Verification items for the finished model (mm, model axes). Face numbers are marked on the shaded views. A direction names the side the tool comes from. Coordinates: 2 decimals unless noted, no trailing zeros. Loops run counter-clockwise (first coordinate to the right, second up) from the corner with the lowest first, then second, coordinate; pieces in that order, holes last.
Q1. Sectioned sample at D-D (z = -3). Enter the section's corners in (x, y), then the cut area to 3 significant figures.
Q2. Sectioned sample at A-A (x = -40.5). Enter the section's corners in (y, z).
Q3. Access from +Z, -Z, +X, -X, +Y, -Y to the whole of each face (thin tool, end or side, straight path). Record for the marked faces 1, 2 and 3.
Q4. Sectioned sample at B-B (y = 0). Count the separate pieces of the cut face and the enclosed holes in it, then the cut area to 3 significant figures.
Q5. Sectioned sample at C-C (x = 44). Enter the section's corners in (y, z), then the cut area to 3 significant figures.
Q6. Go/stop test with flat-tipped pins: P1, Ø0.5, axis at y = -12, z = 1.5, coming from the +X side; P2, Ø23.5, axis at x = -36, y = -9.5, coming from the -Z side; P3, Ø5, axis at x = -40.5, z = -4, coming from the -Y side; P4, Ø4, axis at y = -8.5, z = -6.5, coming from the +X side. Record where each tip stops, or that it passes through.
Q7. Material ranges on probe 1 along Z at (x, y) = (-41, -22); probe 2 along Y at (x, z) = (11, -2.5); probe 3 along Y at (x, z) = (-40.5, 1.9), recorded low to high.
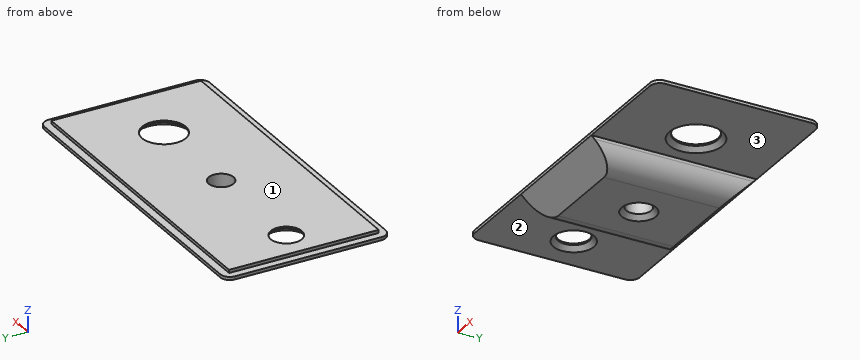
```python
from build123d import *

# Parameters (mm, degrees)
F0_W            = 106
F0_H            = 53
F1_DEPTH        = 1
F2_W            = 101
F2_H            = 48
F3_DEPTH        = 1
F4_R            = 3
F6_D            = 14
F6_CSINK_D      = 17
F6_CSINK_ANGLE  = 90
F7_D            = 10
F7_CSINK_D      = 13
F7_CSINK_ANGLE  = 90
F8_W            = 40
F8_H            = 53
F9_DEPTH        = 8
F11_D           = 8
F11_CSINK_D     = 11
F11_CSINK_ANGLE = 90
F12_SIZE        = 8
F13_R           = 7


with BuildPart() as f1:
    # F0 (on Top) → F1 (new body)
    with BuildSketch(Plane.XY):
        Rectangle(F0_W, F0_H)
    extrude(amount=F1_DEPTH)

    # F2 (on face) → F3 (join)
    with BuildSketch(Plane.XY.offset(1)):
        Rectangle(F2_W, F2_H)
    extrude(amount=F3_DEPTH)

    # F4
    f4_edges = [f1.edges().sort_by_distance(p)[0] for p in [
        (-53, -26.5, 0.5),
        (53, -26.5, 0.5),
        (53, 26.5, 0.5),
        (-53, 26.5, 0.5),
    ]]
    fillet(f4_edges, radius=F4_R)

    # F6 (through all)
    with Locations(Plane(origin=(0, 0, 0), x_dir=(1, 0, 0), z_dir=(0, 0, -1))):
        with Locations((29, 0)):
            CounterSinkHole(F6_D / 2, F6_CSINK_D / 2, counter_sink_angle=F6_CSINK_ANGLE)

    # F7 (through all)
    with Locations(Plane(origin=(0, 0, 0), x_dir=(1, 0, 0), z_dir=(0, 0, -1))):
        with Locations((-40.5, 0)):
            CounterSinkHole(F7_D / 2, F7_CSINK_D / 2, counter_sink_angle=F7_CSINK_ANGLE)

    # F8 (on face) → F9 (join)
    with BuildSketch(Plane(origin=(0, 0, 0), x_dir=(1, 0, 0), z_dir=(0, 0, -1))):
        with Locations((-3.5, 0)):
            Rectangle(F8_W, F8_H)
    extrude(amount=F9_DEPTH)

    # F11 (through all)
    with Locations(Plane(origin=(0, 0, -8), x_dir=(1, 0, 0), z_dir=(0, 0, -1))):
        with Locations((-3.5, 0)):
            CounterSinkHole(F11_D / 2, F11_CSINK_D / 2, counter_sink_angle=F11_CSINK_ANGLE)

    # F12
    f12_edges = [f1.edges().sort_by_distance(p)[0] for p in [
        (-3.5, 26.5, -8),
        (-3.5, -26.5, -8),
    ]]
    chamfer(f12_edges, length=F12_SIZE)

    # F13
    f13_edges = [f1.edges().sort_by_distance(p)[0] for p in [
        (-23.5, 0, -8),
        (16.5, 0, -8),
    ]]
    fillet(f13_edges, radius=F13_R)


solid = f1.part
```
Geometry check:
1. outline: (-23.21, -23.5) - (16.21, -23.5) - (16.21, 23.5) - (-23.21, 23.5) - close; hole circle Ø8 at (-3.5, 0)
1. area: 1,800 mm2
2. outline: (-26.5, 0) - (-6.5, 0) - (-5, 1.5) - (-5, 2) - (-24, 2) - (-24, 1) - (-26.5, 1) - close; (5, 1.5) - (6.5, 0) - (26.5, 0) - (26.5, 1) - (24, 1) - (24, 2) - (5, 2) - close
3. face 1: +Z, +X, -X, +Y, -Y
3. face 2: -Z, -X, +Y, -Y
3. face 3: -Z, +X, +Y, -Y
4. separate pieces: 4
4. enclosed holes: 0
4. area: 371 mm2
5. outline: (-26.5, 0) - (26.5, 0) - (26.5, 1) - (24, 1) - (24, 2) - (-24, 2) - (-24, 1) - (-26.5, 1) - close
5. area: 101 mm2
6. P1: stops at x = 50.5
6. P2: stops at z = 0
6. P3: passes through
6. P4: stops at x = 15.56
7. probe 1: z = 0 to 2
7. probe 2: y = -24 to 24
7. probe 3: y = -24 to -5, 5 to 24
